Read the model definition and answer for the solid it produces. Units are mm, in the model's axes. A direction names the side the tool comes from. Give positions to 0.01 mm unless a question says otherwise; leave off trailing zeros. Write each loop counter-clockwise with the first axis right and the second up, starting at its lowest first coordinate (ties: lowest second). Pieces come first, ordered by that corner, then holes. Notation, with made-up numbers: M -21.75,71 L 26.25,71 A10 ccw 26.25,79 Z; hole C 74,-9 d4. An arc over 180 degrees is marked long. Put each result on its own line as item: value.
from build123d import *

# Parameters (mm, degrees)
BOSS_EXTRUDE1_DEPTH  = 1.5748
SKETCH3_W            = 66.47
SKETCH3_H            = 5.335951997
BOSS_EXTRUDE2_DEPTH  = 1.575
SKETCH4_W            = 66.47
SKETCH4_H            = 0.5
CUT_EXTRUDE1_DEPTH   = 134.633133513
M2_CLEARANCE_HOLE1_D = 2.2
SKETCH5_W            = 5
SKETCH5_H            = 51.15
BOSS_EXTRUDE3_DEPTH  = 1.575
SKETCH6_W            = 24.5
SKETCH6_H            = 2.5
CUT_EXTRUDE2_DEPTH   = 134.633133513


with BuildPart() as part:
    # BPR2 PCB Outline → Boss-Extrude1 (new body)
    with BuildSketch(Plane.XY):
        with BuildLine():
            Line((114.542984325, 6.620432961), (102.642984325, 6.620432961))
            Line((102.642984325, 6.620432961), (82.642984325, 6.620432961))
            Line((82.642984325, 6.620432961), (49.072984325, 6.620432961))
            Line((49.072984325, 6.620432961), (49.072984325, 66.120432961))
            ThreePointArc((49.072984325, 66.120432961), (49.365877543, 66.827539743), (50.072984325, 67.120432961))
            Line((50.072984325, 67.120432961), (114.542984325, 67.120432961))
            ThreePointArc((114.542984325, 67.120432961), (115.250091106, 66.827539743), (115.542984325, 66.120432961))
            Line((115.542984325, 66.120432961), (115.542984325, 7.620432961))
            ThreePointArc((115.542984325, 7.620432961), (115.250091106, 6.91332618), (114.542984325, 6.620432961))
        make_face()
    extrude(amount=-BOSS_EXTRUDE1_DEPTH)

    # Sketch3 → Boss-Extrude2 (add)
    with BuildSketch(Plane.XY):
        with Locations((82.307984325, 9.288408959)):
            Rectangle(SKETCH3_W, SKETCH3_H)
    extrude(amount=-BOSS_EXTRUDE2_DEPTH)

    # Sketch4 → Cut-Extrude1 (cut, through all)
    with BuildSketch(Plane.XY):
        with Locations((82.307984325, 6.870432961)):
            Rectangle(SKETCH4_W, SKETCH4_H)
    extrude(amount=-CUT_EXTRUDE1_DEPTH, mode=Mode.SUBTRACT)

    # M2 Clearance Hole1 (through all)
    with Locations(Plane(origin=(32.762906477, 104.007481373, -6.5748), x_dir=(1, 0, 0), z_dir=(0, 0, -1))):
        with Locations((18.060077848, 88.112048412), (18.060077848, 46.962048412), (81.030077848, 46.962048412), (81.030077848, 64.537048412), (81.030077848, 88.112048412), (81.030077848, 72.537048412)):
            Hole(M2_CLEARANCE_HOLE1_D / 2)

    # Sketch5 → Boss-Extrude3 (add)
    with BuildSketch(Plane.XY):
        with Locations((46.572984325, 36.470432961)):
            Rectangle(SKETCH5_W, SKETCH5_H)
    extrude(amount=-BOSS_EXTRUDE3_DEPTH)

    # Sketch6 → Cut-Extrude2 (cut, through all)
    with BuildSketch(Plane.XY):
        with Locations((97.792984325, 65.870432961)):
            Rectangle(SKETCH6_W, SKETCH6_H)
    extrude(amount=-CUT_EXTRUDE2_DEPTH, mode=Mode.SUBTRACT)


solid = part.part
(1) Straight lines are drawn through the part: line 1 along Y through (x, z) = (51, -0.3); line 2 along Y through (x, z) = (90, -0.2); line 3 along Y through (x, z) = (49, -1.35). For each, find the intervals that lie inside material, in ascending order. Write a range as from..to.
Result:
line 1: y = 7.12..14.81, 16.98..55.96, 58.13..67.12
line 2: y = 7.12..64.62
line 3: y = 10.9..62.05
(2) Section B-B on z = -1.25 is taken. Determine the outline of the cut face in (x, y), and give its area (3 significant figures).
Result:
outline: M 44.07,10.9 L 49.07,10.9 L 49.07,7.12 L 115.54,7.12 L 115.54,66.12 A1 ccw 114.54,67.12 L 110.04,67.12 L 110.04,64.62 L 85.54,64.62 L 85.54,67.12 L 50.07,67.12 A1 ccw 49.07,66.12 L 49.07,62.05 L 44.07,62.05 Z; hole C 50.82,15.9 d2.2; hole C 50.82,57.05 d2.2; hole C 113.79,15.9 d2.2; hole C 113.79,31.47 d2.2; hole C 113.79,39.47 d2.2; hole C 113.79,57.05 d2.2
area: 4,160 mm²
(3) Which of the six approach directions +Z, -Z, +X, -X, +Y, -Y give full straight-line access (tool end or side, diameter ignored) to faces 1 (the face through (98, 64.62, -1)), 2 (the face through (47, 10.895, -1)), 3 (the face through (47, 62.045, -1))?
Result:
face 1: +Z, -Z, +Y
face 2: +Z, -Z, -X, -Y
face 3: +Z, -Z, -X, +Y
(4) Given pin 1 Ø0.5 at (x, z) = (98.5, -0.5) entering from +Y; pin 2 Ø0.5 at (y, z) = (66, -0.5) entering from -X; pin 3 Ø0.5 at (y, z) = (66.5, -1) entering from +X, each flat-ended and moving along its own axis, determine where each tip first touches the part or whether it passes through.
Result:
pin 1: stops at y = 64.62
pin 2: stops at x = 49.07
pin 3: stops at x = 115.53
(5) For a pull along Y with two mould halves and no side action, classify faces 4 (the face through (114.666, 32.14, -0.776)), 5 (the face through (112, 67.12, -1)), 6 (the face through (51.922, 15.847, -0.776)), 7 (the face through (82, 7.12, -1)) as +Y half, -Y half, draft (parallel to the pull), parting line (faces both ways), or undercut.
Result:
face 4: undercut
face 5: +Y half
face 6: undercut
face 7: -Y half
